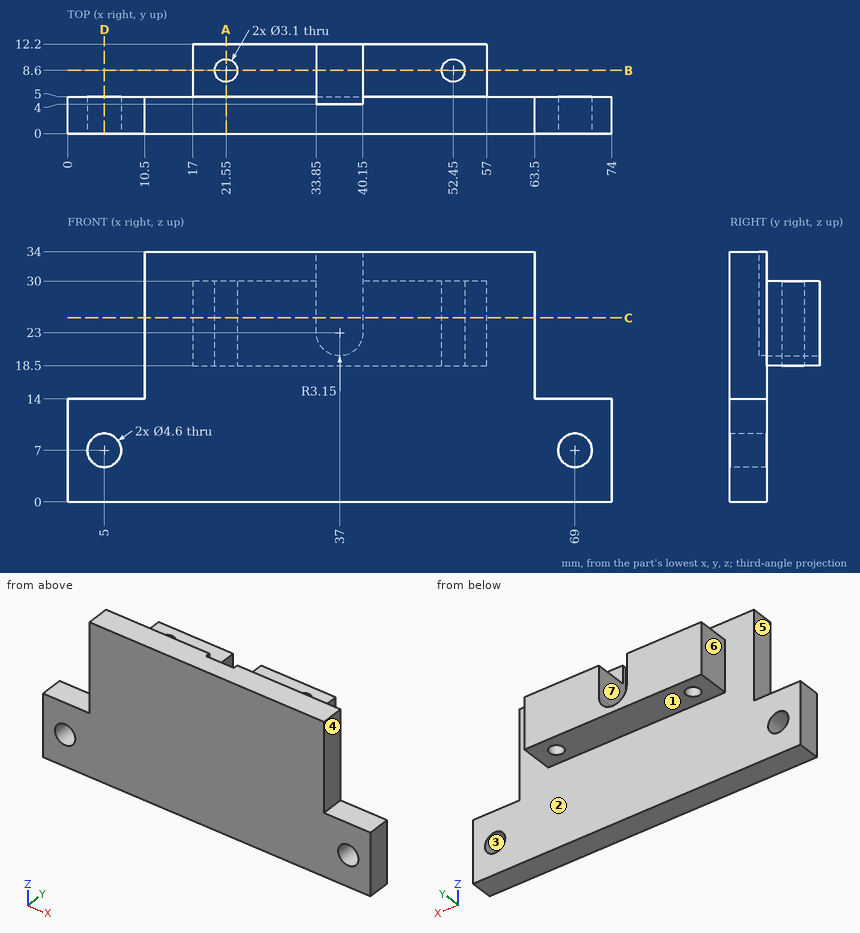
Verification items for this drawing (mm, ordinates from the low corner). A direction names the side the tool comes from. Coordinates: 2 decimals unless noted, no trailing zeros. Write each loop counter-clockwise with the first axis right and the second up, starting at its lowest first coordinate (ties: lowest second). Pieces come first, ordered by that corner, then holes. Notation, with made-up numbers: M -2,-39.75 L 14,-39.75 A30 ccw 14,-12.75 Z; hole C -23,-34 d10. An arc over 180 degrees is marked long. Use one line per item in the form item = value. Start each with the question number.
1) Section check D-D on x = 5. Enter the section's corners in (y, z), and give its area (3 significant figures).
2) Section check A-A on x = 21.55. Enter the section's corners in (y, z), and give its area (3 significant figures).
3) Go/stop test with flat-tipped pins: pin 1 Ø4 at (x, y) = (21.55, 8.6) entering from +Z; pin 2 Ø6.5 at (y, z) = (6.5, 31) entering from +X; pin 3 Ø1.5 at (x, y) = (31, 10.5) entering from -Z. Record where each tip stops, or that it passes through.
4) Section check C-C on z = 25. Enter the section's corners in (x, y).
5) Thickness scan on probe 1 along X at (y, z) = (3.7, 7); probe 2 along Y at (x, z) = (52.45, 24); probe 3 along X at (y, z) = (7, 23). Record the ranges inside material, lowest first. Write a range as from..to.
6) Set-up check for the marked faces 4, 5, 6 and 7: record each of +Z, -Z, +X, -X, +Y, -Y from which the full face is reachable in a straight line by a thin tool's end or side.
7) Release check for a two-part mould opening along Z. For the marked faces 1, 2 and 3 record: pulls with the +Z half, pulls with the -Z half, needs draft (parallel to the pull), parting line crosses it, or undercut.
8) Section check B-B on y = 8.6. Enter the section's corners in (x, z), and give its area (3 significant figures).
Responses:
q1.outline = M 0,0 L 5,0 L 5,4.7 L 0,4.7 Z; M 0,9.3 L 5,9.3 L 5,14 L 0,14 Z
q1.area = 47.0 mm2
q2.outline = M 0,0 L 5,0 L 5,18.5 L 7.05,18.5 L 7.05,30 L 5,30 L 5,34 L 0,34 Z; M 10.15,18.5 L 12.2,18.5 L 12.2,30 L 10.15,30 Z
q2.area = 217 mm2
q3.pin_1 = 30
q3.pin_2 = 63.5
q3.pin_3 = 18.5
q4.outline = M 10.5,0 L 63.5,0 L 63.5,5 L 57,5 L 57,12.2 L 40.15,12.2 L 40.15,4 L 33.85,4 L 33.85,12.2 L 17,12.2 L 17,5 L 10.5,5 Z; hole C 21.55,8.6 d3.1; hole C 52.45,8.6 d3.1
q5.probe_1 = 0..2.7, 7.3..66.7, 71.3..74
q5.probe_2 = 0..7.05, 10.15..12.2
q5.probe_3 = 17..33.85, 40.15..57
q6.face_4 = +Z, +X, +Y, -Y
q6.face_5 = +Z, -X, +Y, -Y
q6.face_6 = +Z, -Z, -X, +Y
q6.face_7 = +Z, +Y
q7.face_1 = pulls with the -Z half
q7.face_2 = needs draft
q7.face_3 = undercut
q8.outline = M 17,18.5 L 20,18.5 L 20,30 L 17,30 Z; M 23.1,18.5 L 50.9,18.5 L 50.9,30 L 40.15,30 L 40.15,23 A3.15 cw 33.85,23 L 33.85,30 L 23.1,30 Z; M 54,18.5 L 57,18.5 L 57,30 L 54,30 Z
q8.area = 329 mm2
